The drawing under review shows one solid part. Ordinate dimensions are in mm from its lowest x, y, z. A direction names the side the tool comes from. Round coordinates to 2 decimals unless told otherwise and drop trailing zeros. Order: outer loops, then holes, each group sorted by start corner. A loop starts at its lowest first (then second) coordinate and runs counter-clockwise, first axis right, second up.
1) Mouldability with a two-part tool opening along Y and no side actions: class the marked faces 1, 2 and 3 as pulls with the +Y half, pulls with the -Y half, needs draft (parallel to the pull), parting line crosses it, or undercut.
2) To check wall thickness, follow L1, parallel to Y at x = 5.5, z = 47.5; L2, parallel to Z at x = 25.5, y = 34.5; L3, parallel to X at y = 66.5, z = 7. State the ranges of each line that lie inside material, in increasing order.
3) Consider section C-C (y = 71). Give the boundary of the cut face in (x, z) (1 decimal).
4) Machinability: for the marked faces 4 and 5, which of the approach directions +Z, -Z, +X, -X, +Y, -Y give a long, thin tool a straight path to every point of the face, cutting with its end or side? Answer none if there is none.
5) Clearance check with flat-ended pins moving along their axes: P1, Ø1, axis at x = 23.5, z = 41, coming from the +Y side; P2, Ø13.5, axis at x = 33.5, y = 37.5, coming from the +Z side. State where each tip first meets the part, or that it passes through.
6) Consider section B-B (x = 19). Give the boundary of the cut face in (y, z), then the cut area to 3 significant figures.
7) Consider section D-D (y = 13). Give the boundary of the cut face in (x, z), then the cut area to 3 significant figures.
8) Consider section A-A (z = 45.5). Give the boundary of the cut face in (x, y).
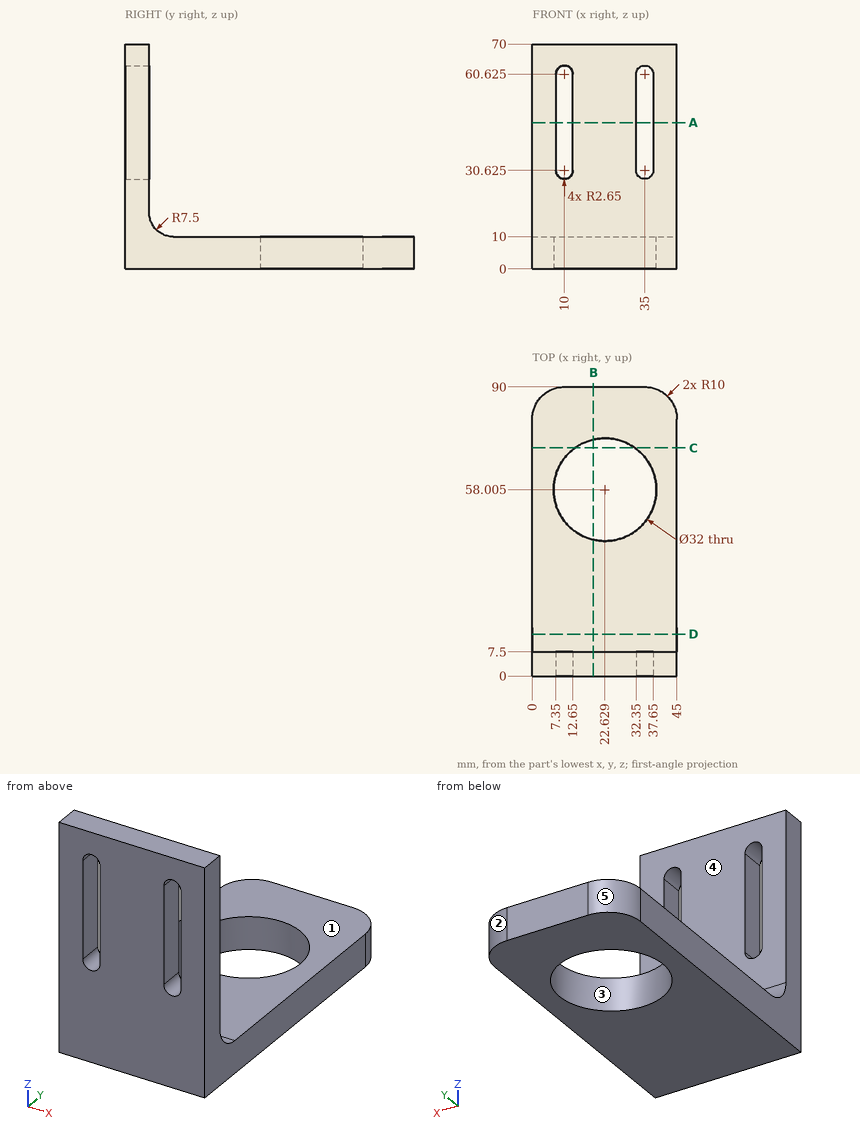
Answer below:
1. face 1: needs draft
1. face 2: pulls with the +Y half
1. face 3: undercut
2. L1: y = 0 to 7.5
2. L2: z = 0 to 10
2. L3: x = 0 to 9.07, 36.19 to 45
3. outline: (0, 0) - (13.3, 0) - (13.3, 10) - (0, 10) - close; (32, 0) - (45, 0) - (45, 10) - (32, 10) - close
4. face 4: +Z, +X, -X, +Y
4. face 5: +Z, -Z, -X, +Y
5. P1: stops at y = 7.5
5. P2: stops at z = 10
6. outline: (0, 0) - (42.42, 0) - (42.42, 10) - (15, 10) arc R7.5 cw to (7.5, 17.5) - (7.5, 70) - (0, 70) - close; (73.59, 0) - (90, 0) - (90, 10) - (73.59, 10) - close
6. area: 1,050 mm2
7. outline: (0, 0) - (45, 0) - (45, 10.27) - (0, 10.27) - close
7. area: 462 mm2
8. outline: (0, 0) - (7.35, 0) - (7.35, 7.5) - (0, 7.5) - close; (12.65, 0) - (32.35, 0) - (32.35, 7.5) - (12.65, 7.5) - close; (37.65, 0) - (45, 0) - (45, 7.5) - (37.65, 7.5) - close
